Autodesk Inventor part; units mm, degrees
ref_plane "YZ Plane" through (0, 0, 0) normal (1, 0, 0) x (0, 1, 0)
ref_plane "XZ Plane" through (0, 0, 0) normal (0, 1, 0) x (-1, 0, 0)
ref_plane "XY Plane" through (0, 0, 0) normal (0, 0, 1) x (1, 0, 0)
sketch "스케치1" plane through (0, 0, 0) normal (0, 1, 0) x (-1, 0, 0)
  line L0 (-2.4, 4.8) -> (2.4, 4.8)
  line L1 (2.4, 4.8) -> (2.4, -4.8)
  line L2 (2.4, -4.8) -> (-2.4, -4.8)
  line L3 (-2.4, -4.8) -> (-2.4, 4.8)
  line L4 (-2.4, 4.8) -> (2.4, -4.8) construction
  line L5 (2.4, 4.8) -> (-2.4, -4.8) construction
  circle A0 centre (0, 0) radius 2.85
  circle A1 centre (0, 0) radius 1.9
  dimension "d0" = 4.8
  dimension "d1" = 9.6
  dimension "d17" = 5.7
  dimension "d18" = 3.8
extrude "돌출1" add sketch "스케치1" along normal blind 0.6 contours L0 L1 A0 L3 | A0 L1 L3 | A0 L1 L2 L3 | A1
sketch "스케치2" plane through (0, 0, 0) normal (0, -1, 0) x (1, 0, 0)
  line L0 (2.4, -4.8) -> (-2.4, -4.8)
  line L1 (2.4, 4.8) -> (2.4, -4.8)
  line L2 (-2.4, 4.8) -> (2.4, 4.8)
  line L3 (-2.4, -4.8) -> (-2.4, 4.8)
  line L4 (2.4, 4.8) -> (3, 4.8)
  line L5 (3, 4.8) -> (3, -4.8)
  line L6 (3, -4.8) -> (2.4, -4.8)
  line L7 (2.4, -4.8) -> (2.4, 4.8)
  line L8 (-2.4, -4.8) -> (-2.4, 4.8)
  line L9 (-2.4, 4.8) -> (-3, 4.8)
  line L10 (-3, 4.8) -> (-3, -4.8)
  line L11 (-3, -4.8) -> (-2.4, -4.8)
  line L12 (-2.4, -4.8) -> (-2.4, 4.8)
  point P0 (0, 0)
  dimension "d4" = 0.6
  dimension "d5" = 0.6
extrude "돌출2" add sketch "스케치2" against normal blind 3.1 contours L1 L4 L5 L6 | L11 L10 L9 L3
extrude "돌출5" add sketch "스케치1" against normal blind 2.5 contours A0 L1 L3 | L3 A0 | A0 L1
properties part number "endcap_4mm_2ea_typeB_ver2_onyx_addon"
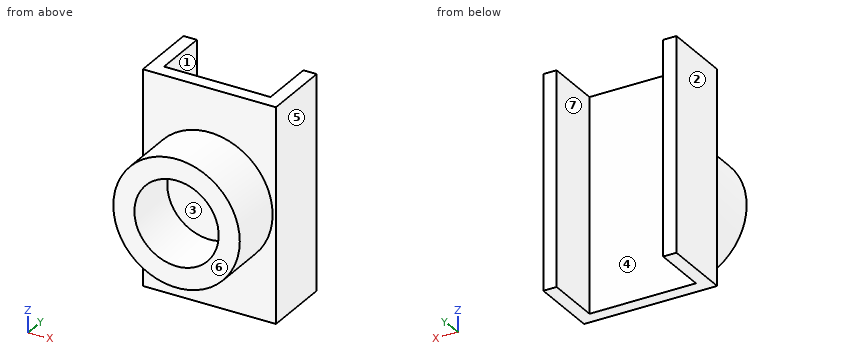
The model under review builds one solid part; all positions refer to its coordinate system, in mm. Face numbers are marked on the shaded views. A direction names the side the tool comes from. Round coordinates to 2 decimals unless told otherwise and drop trailing zeros. Loops run counter-clockwise (first coordinate to the right, second up) from the corner with the lowest first, then second, coordinate; pieces in that order, holes last. Notation, with made-up numbers: (72.25, 84) - (102.25, 84) arc R20 ccw to (102.25, 106) - close; hole circle Ø2 at (-18.75, -15). An arc over 180 degrees is marked (long way). Use CSV: the item, a comma, the result in double quotes.
(1) Take a section at D-D, the plane y = -1.75. Give the boundary of the cut face in (x, z), plus the area to 3 significant figures.
Working result:
outline,"circle Ø5.7 at (0, 0); hole circle Ø3.8 at (0, 0)"
area,"14.2 mm^2"
(2) Machinability: for the marked faces 1, 2 and 3, which of the approach directions +Z, -Z, +X, -X, +Y, -Y give a long, thin tool a straight path to every point of the face, cutting with its end or side? Answer none if there is none.
Working result:
face 1,"+Z, -Z, +Y"
face 2,"+Z, -Z, -X, +Y, -Y"
face 3,"-Y"
(3) For line 1 (Z direction, x = 0, y = -0.7); line 2 (X direction, y = 0.8, z = -1.5); line 3 (Y direction, x = -1.9, z = -2), list the stretches that pass through material, from the lowest coordinate up.
Working result:
line 1,"z = -2.85 to -1.9, 1.9 to 2.85"
line 2,"x = -3 to -2.4, 2.4 to 3"
line 3,"y = -2.5 to 0.6"
(4) Take a section at B-B, the plane z = 4. Give the boundary of the cut face in (x, y).
Working result:
outline,"(-3, 0) - (3, 0) - (3, 3.1) - (2.4, 3.1) - (2.4, 0.6) - (-2.4, 0.6) - (-2.4, 3.1) - (-3, 3.1) - close"
(5) Clearance check with a flat-ended pin moving along its axis: P1, Ø2, axis at x = -2, y = 2.5, coming from the -Z side. State where the tip first meets the part, or that it passes through.
Working result:
P1,"stops at z = -4.8"
(6) The part is to be moulded in two halves that separate along X. For the marked faces 4, 5, 6 and 7, say which applies: pulls with the +X half, pulls with the -X half, needs draft (parallel to the pull), parting line crosses it, or undercut.
Working result:
face 4,"undercut"
face 5,"pulls with the +X half"
face 6,"needs draft"
face 7,"undercut"
(7) Take a section at A-A, the plane y = 0.75. Give the boundary of the cut face in (x, z), plus the area to 3 significant figures.
Working result:
outline,"(-3, -4.8) - (-2.4, -4.8) - (-2.4, 4.8) - (-3, 4.8) - close; (2.4, -4.8) - (3, -4.8) - (3, 4.8) - (2.4, 4.8) - close"
area,"11.5 mm^2"
(8) Take a section at C-C, the plane x = 0. Give the boundary of the cut face in (y, z), plus the area to 3 significant figures.
Working result:
outline,"(-2.5, -2.85) - (0, -2.85) - (0, -4.8) - (0.6, -4.8) - (0.6, 4.8) - (0, 4.8) - (0, 2.85) - (-2.5, 2.85) - (-2.5, 1.9) - (0, 1.9) - (0, -1.9) - (-2.5, -1.9) - close"
area,"10.5 mm^2"
